Design review of the part built by this model. Coordinates are the model's own, in mm. Face numbers are marked on the shaded views. A direction names the side the tool comes from. Coordinates: 2 decimals unless noted, no trailing zeros. Loops run counter-clockwise (first coordinate to the right, second up) from the corner with the lowest first, then second, coordinate; pieces in that order, holes last.
Q1. Add section B-B on z = 0. Give the boundary of the cut face in (x, y).
Q2. Add section A-A on x = 85. Give the boundary of the cut face in (y, z), and give its area (3 significant figures).
Q3. Add section D-D on x = 41. Give the boundary of the cut face in (y, z).
Q4. Wall thickness on probe 1 along Z at (x, y) = (0, -5.3); probe 2 along Z at (x, y) = (85, -13.8); probe 3 along Z at (x, y) = (30.5, -3.25): over which ranges is each line inside the solid? List them lowest first.
Q5. Add section C-C on x = 0. Give the boundary of the cut face in (y, z).
Q6. Machinability: for the marked faces 1, 2 and 3, which of the approach directions +Z, -Z, +X, -X, +Y, -Y give a long, thin tool a straight path to every point of the face, cutting with its end or side? Answer none if there is none.
Q7. For P1, Ø4, axis at x = 83, y = -12, coming from the -Z side; P2, Ø9.5, axis at x = 85, z = 0, coming from the -Y side; P3, Ø1, axis at x = 43, z = -8, coming from the +Y side; P4, Ø5, axis at x = 55, z = 3, coming from the -Y side, all flat-tipped, find the tip position at first contact; note any pin that passes through.
```python
from build123d import *

# Parameters (mm, degrees)
F0_R     = 6
F1_DEPTH = 25
F3_DEPTH = 317.5
F4_R     = 2.54


with BuildPart() as f1:
    # F0 (on Front) → F1 (new body)
    with BuildSketch(Plane.XZ):
        with BuildLine():
            ThreePointArc((12.2088000741, -8), (13.9867667719, -4.1743448012), (14.59639679, 0))
            ThreePointArc((14.59639679, 0), (13.9867667719, 4.1743448012), (12.2088000741, 8))
            ThreePointArc((12.2088000741, 8), (-14.59639679, 0), (12.2088000741, -8))
        make_face()
        Circle(F0_R, mode=Mode.SUBTRACT)
        with BuildLine():
            ThreePointArc((12.2088000741, 8), (13.9867667719, 4.1743448012), (14.59639679, 0))
            ThreePointArc((14.59639679, 0), (13.9867667719, -4.1743448012), (12.2088000741, -8))
            Line((12.2088000741, -8), (79, -8))
            ThreePointArc((79, -8), (75, 0), (79, 8))
            Line((79, 8), (12.2088000741, 8))
        make_face()
        with BuildLine():
            ThreePointArc((95, 0), (89.472135955, 8.94427191), (79, 8))
            ThreePointArc((79, 8), (75, 0), (79, -8))
            ThreePointArc((79, -8), (89.472135955, -8.94427191), (95, 0))
        make_face()
        with Locations((85, 0)):
            Circle(F0_R, mode=Mode.SUBTRACT)
    extrude(amount=F1_DEPTH)

    # F2 (on Top) → F3 (intersect, symmetric)
    with BuildSketch(Plane.XY):
        Polygon((20, 0), (-14.4787151366, 0), (-14.4787151366, -9), (19.2126020283, -9), (70.2541384048, -18), (94.5431698973, -18), (94.5431698973, -9), (71.0415363766, -9), align=None)
    extrude(amount=F3_DEPTH, both=True, mode=Mode.INTERSECT)

    # F4
    f4_edges = [f1.edges().sort_by_distance(p)[0] for p in [
        (-6, -9, 0),
        (79, -18, 0),
        (-6, 0, 0),
        (79, -9, 0),
    ]]
    fillet(f4_edges, radius=F4_R)


solid = f1.part
```
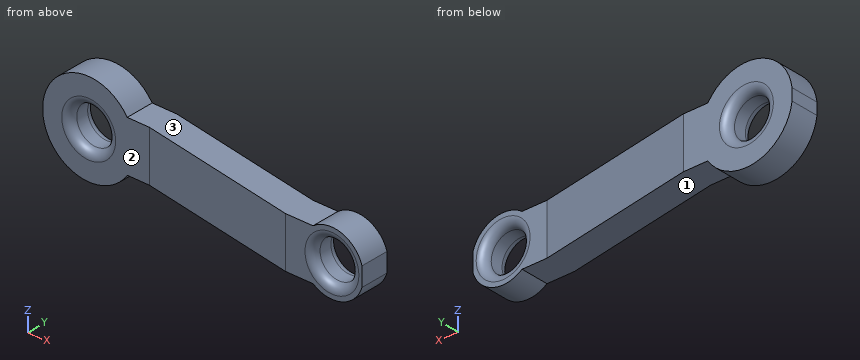
Entries:
1. outline: (-14.48, -9) - (-8.54, -9) arc R2.54 ccw to (-6, -6.46) - (-6, -2.54) arc R2.54 ccw to (-8.54, 0) - (-14.48, 0) - close; (6, -6.46) arc R2.54 ccw to (8.54, -9) - (19.21, -9) - (70.25, -18) - (76.46, -18) arc R2.54 ccw to (79, -15.46) - (79, -11.54) arc R2.54 ccw to (76.46, -9) - (71.04, -9) - (20, 0) - (8.54, 0) arc R2.54 ccw to (6, -2.54) - close; (91, -15.46) arc R2.54 ccw to (93.54, -18) - (94.54, -18) - (94.54, -9) - (93.54, -9) arc R2.54 ccw to (91, -11.54) - close
2. outline: (-18, -10) - (-9, -10) - (-9, -8.54) arc R2.54 ccw to (-11.54, -6) - (-15.46, -6) arc R2.54 ccw to (-18, -8.54) - close; (-18, 8.54) arc R2.54 ccw to (-15.46, 6) - (-11.54, 6) arc R2.54 ccw to (-9, 8.54) - (-9, 10) - (-18, 10) - close
2. area: 66.5 mm2
3. outline: (-12.84, -8) - (-3.7, -8) - (-3.7, 8) - (-12.84, 8) - close
4. probe 1: z = -14.6 to -6, 6 to 14.6
4. probe 2: z = -10 to -6, 6 to 10
4. probe 3: z = -8 to 8
5. outline: (-9, -14.6) - (0, -14.6) - (0, -8.54) arc R2.54 ccw to (-2.54, -6) - (-6.46, -6) arc R2.54 ccw to (-9, -8.54) - close; (-9, 8.54) arc R2.54 ccw to (-6.46, 6) - (-2.54, 6) arc R2.54 ccw to (0, 8.54) - (0, 14.6) - (-9, 14.6) - close
6. face 1: -Z, +Y, -Y
6. face 2: +Z, -Z, -X, -Y
6. face 3: +Z, +Y, -Y
7. P1: stops at z = -10
7. P2: passes through
7. P3: stops at y = -3.97
7. P4: stops at y = -15.75
